from build123d import *

# Parameters (mm, degrees)
SKETCH_1_R          = 4.85
EXTRUDE_1_DEPTH     = 6.8
SKETCH_2_R          = 4
CUT_EXTRUDE_1_DEPTH = 0.5
CHAMFER_1_SIZE      = 0.5
EXTRUDE_2_DEPTH     = 0.8
FILLET_1_R          = 0.4
SKETCH_4_R          = 4.65
EXTRUDE_3_DEPTH     = 0.2


with BuildPart() as part:
    # Эскиз1 → Бобышка-Вытянуть1 (new body)
    with BuildSketch(Plane.XY):
        Circle(SKETCH_1_R)
    extrude(amount=EXTRUDE_1_DEPTH)

    # Эскиз2 → Вырез-Вытянуть1 (cut)
    with BuildSketch(Plane.XY.offset(6.8)):
        Circle(SKETCH_2_R)
    extrude(amount=-CUT_EXTRUDE_1_DEPTH, mode=Mode.SUBTRACT)

    # Фаска1
    chamfer_1_edges = [part.edges().sort_by_distance(p)[0] for p in [
        (-4, 0, 6.8),
    ]]
    chamfer(chamfer_1_edges, length=CHAMFER_1_SIZE - 0.0001)  # a hair under: the kernel refuses the full size

    # Эскиз3 → Бобышка-Вытянуть2 (add)
    with BuildSketch(Plane.XY.offset(6.3)):
        with BuildLine():
            Line((-1.695763296, 2), (-1.395763296, 2))
            ThreePointArc((-1.395763296, 2), (-0.971499227, 1.824264069), (-0.795763296, 1.4))
            Line((-0.795763296, 1.4), (-0.795763296, -1.4))
            ThreePointArc((-0.795763296, -1.4), (-0.971499227, -1.824264069), (-1.395763296, -2))
            Line((-1.395763296, -2), (-1.695763296, -2))
            ThreePointArc((-1.695763296, -2), (-2.120027365, -1.824264069), (-2.295763296, -1.4))
            Line((-2.295763296, -1.4), (-2.295763296, 1.4))
            ThreePointArc((-2.295763296, 1.4), (-2.120027365, 1.824264069), (-1.695763296, 2))
        make_face()
        with BuildLine():
            Line((0.795763296, 1.4), (0.795763296, -1.4))
            ThreePointArc((0.795763296, -1.4), (0.971499227, -1.824264069), (1.395763296, -2))
            Line((1.395763296, -2), (1.695763296, -2))
            ThreePointArc((1.695763296, -2), (2.120027365, -1.824264069), (2.295763296, -1.4))
            Line((2.295763296, -1.4), (2.295763296, 1.4))
            ThreePointArc((2.295763296, 1.4), (2.120027365, 1.824264069), (1.695763296, 2))
            Line((1.695763296, 2), (1.395763296, 2))
            ThreePointArc((1.395763296, 2), (0.971499227, 1.824264069), (0.795763296, 1.4))
        make_face()
    extrude(amount=EXTRUDE_2_DEPTH)

    # Скругление1
    fillet_1_edges = [part.edges().sort_by_distance(p)[0] for p in [
        (-2.120027365, -1.824264069, 7.1),
        (-1.545763296, -2, 7.1),
        (-0.971499227, -1.824264069, 7.1),
        (-0.795763296, 0, 7.1),
        (-0.971499227, 1.824264069, 7.1),
        (-1.545763296, 2, 7.1),
        (-2.120027365, 1.824264069, 7.1),
        (-2.295763296, 0, 7.1),
        (2.120027365, 1.824264069, 7.1),
        (1.545763296, 2, 7.1),
        (0.971499227, 1.824264069, 7.1),
        (0.795763296, 0, 7.1),
        (0.971499227, -1.824264069, 7.1),
        (1.545763296, -2, 7.1),
        (2.120027365, -1.824264069, 7.1),
        (2.295763296, 0, 7.1),
    ]]
    fillet(fillet_1_edges, radius=FILLET_1_R)

    # Эскиз4 → Бобышка-Вытянуть3 (add)
    with BuildSketch(Plane(origin=(0, 0, 0), x_dir=(-1, 0, 0), z_dir=(0, 0, -1))):
        with Locations(Location((0, 0, 0), (0, 0, 180))):
            Circle(SKETCH_4_R)
    extrude(amount=EXTRUDE_3_DEPTH)


solid = part.part
Read the model definition and answer for the solid it produces. Units are mm, in the model's axes. Coordinates: 2 decimals unless noted, no trailing zeros. Loops run counter-clockwise (first coordinate to the right, second up) from the corner with the lowest first, then second, coordinate; pieces in that order, holes last.
Q1. Each of these flat-tipped pins is pushed along its axis until it touches: pin 1 Ø1.5 at (y, z) = (1, 1.5) entering from +X; pin 2 Ø4 at (x, y) = (4, -1) entering from +Z. Where does it stop, or does it pass through?
Q2. The part is cut by section D-D on z = 2.5. Write down the section's boundary in (x, y), and give its area (3 significant figures).
Q3. The mould has two halves that part along Y. Classify faces 1 (the face through (4.626, 1.457, 3.352)), 2 (the face through (0, 0, -0.2)), 3 (the face through (0, 0, 6.3)): +Y half, -Y half, draft (parallel to the pull), parting line (faces both ways), or undercut.
Q4. Consider probe 1 along Z at (x, y) = (2.25, 4.25); probe 2 along Z at (x, y) = (-1, 2.75); probe 3 along Y at (x, z) = (-3.5, 6.5). Determine where each line is inside the solid, lowest interval first.
Q5. The part is cut by section B-B on z = 6.5. Write down the section's boundary in (x, y), and give its area (3 significant figures).
Results below:
1. pin 1: stops at x = 4.84
1. pin 2: stops at z = 7.09
2. outline: circle Ø9.7 at (0, 0)
2. area: 73.9 mm2
3. face 1: parting line
3. face 2: draft
3. face 3: undercut
4. probe 1: z = 0 to 6.8
4. probe 2: z = -0.2 to 6.3
4. probe 3: y = -3.36 to -2.32, 2.32 to 3.36
5. outline: circle Ø9.7 at (0, 0); (-2.3, -1.4) arc R0.6 ccw to (-1.7, -2) - (-1.4, -2) arc R0.6 ccw to (-0.8, -1.4) - (-0.8, 1.4) arc R0.6 ccw to (-1.4, 2) - (-1.7, 2) arc R0.6 ccw to (-2.3, 1.4) - close; (0.8, -1.4) arc R0.6 ccw to (1.4, -2) - (1.7, -2) arc R0.6 ccw to (2.3, -1.4) - (2.3, 1.4) arc R0.6 ccw to (1.7, 2) - (1.4, 2) arc R0.6 ccw to (0.8, 1.4) - close; hole circle Ø8.4 at (0, 0)
5. area: 29.9 mm2
